from build123d import *

# Parameters (mm, degrees)
F1_DEPTH = 57.15
F2_W     = 25.4
F2_H     = 25.4
F3_DEPTH = 19.05


with BuildPart() as f1:
    # F0 (on Top) → F1 (new body)
    with BuildSketch(Plane.XY):
        Polygon((0, 50.8), (0, 0), (83.82, 0), (83.82, 19.05), (39.37, 19.05), (39.37, 38.1), (19.05, 38.1), (19.05, 50.8), align=None)
    extrude(amount=-F1_DEPTH)

    # F2 (on face) → F3 (cut, through all)
    with BuildSketch(Plane(origin=(0, 19.05, 0), x_dir=(-1, 0, 0), z_dir=(0, 1, 0))):
        with Locations((-71.12, -44.45)):
            Rectangle(F2_W, F2_H)
    extrude(amount=-F3_DEPTH, mode=Mode.SUBTRACT)


solid = f1.part
Check sheet for the modelled part. Datum: model origin and axes. Units: mm. A direction names the side the tool comes from. Round coordinates to 2 decimals unless told otherwise and drop trailing zeros. Loops run counter-clockwise (first coordinate to the right, second up) from the corner with the lowest first, then second, coordinate; pieces in that order, holes last. Notation, with made-up numbers: M 28,-8 L 56,-8 A31 cw 56,26 Z; hole C 14.25,-23 d3. An arc over 180 degrees is marked long. One line per item, written item: value.
(1) Depth check by flat-ended pin: pin 1 Ø5 at (y, z) = (32, -51) entering from +X; pin 2 Ø12 at (x, y) = (23, 28.5) entering from +Z; pin 3 Ø14 at (y, z) = (46.5, -25) entering from +X; pin 4 Ø10 at (x, z) = (29, -37.5) entering from +Y. Enter the tip coordinate at first touch or a pass-through.
Computed values:
pin 1: stops at x = 39.37
pin 2: stops at z = 0
pin 3: stops at x = 19.05
pin 4: stops at y = 38.1
(2) Thickness scan on line 1 (X direction, y = 34, z = -4.5); line 2 (X direction, y = 6.5, z = -41); line 3 (Y direction, x = 55, z = -6.5). Record the ranges inside material, lowest first.
Computed values:
line 1: x = 0 to 39.37
line 2: x = 0 to 58.42
line 3: y = 0 to 19.05
(3) Sectioned sample at D-D, the plane z = -6.5. Record the cut outline in (x, y), then the cut area to 3 significant figures.
Computed values:
outline: M 0,0 L 83.82,0 L 83.82,19.05 L 39.37,19.05 L 39.37,38.1 L 19.05,38.1 L 19.05,50.8 L 0,50.8 Z
area: 2,590 mm^2
(4) Sectioned sample at C-C, the plane x = 61.5. Record the cut outline in (y, z), then the cut area to 3 significant figures.
Computed values:
outline: M 0,-31.75 L 19.05,-31.75 L 19.05,0 L 0,0 Z
area: 605 mm^2
(5) Sectioned sample at A-A, the plane y = 8. Record the cut outline in (x, z).
Computed values:
outline: M 0,-57.15 L 58.42,-57.15 L 58.42,-31.75 L 83.82,-31.75 L 83.82,0 L 0,0 Z
(6) Sectioned sample at B-B, the plane z = -38. Record the cut outline in (x, y).
Computed values:
outline: M 0,0 L 58.42,0 L 58.42,19.05 L 39.37,19.05 L 39.37,38.1 L 19.05,38.1 L 19.05,50.8 L 0,50.8 Z
(7) Access from +Z, -Z, +X, -X, +Y, -Y to the whole of each face (thin tool, end or side, straight path). Record for faces 1 (the face through (58.42, 10, -45)), 2 (the face through (19.05, 44, -28)), 3 (the face through (22, 20, -57.15)).
Computed values:
face 1: -Z, +X, +Y, -Y
face 2: +Z, -Z, +X, +Y
face 3: -Z, +X, -X, +Y, -Y
